from build123d import *

# Parameters (mm, degrees)
SKETCH1_R           = 6.25
SKETCH1_R_2         = 2.6
SKETCH1_R_3         = 6
SKETCH1_W           = 7.5
SKETCH1_H           = 50.316251501
BOSS_EXTRUDE1_DEPTH = 6.5
FILLET1_R           = 10


with BuildPart() as part:
    # Sketch1 → Boss-Extrude1 (new body)
    # profile 1 of 3: a face of its own
    with BuildSketch(Plane(origin=(0, 0, 0), x_dir=(1, 0, 0), z_dir=(0, 1, 0))):
        with Locations((0, 60)):
            Circle(SKETCH1_R)
        with Locations(Location((0, 60, 0), (0, 0, 90))):
            Circle(SKETCH1_R_2, mode=Mode.SUBTRACT)
    # profile 2 of 3: a face of its own
    with BuildSketch(Plane(origin=(0, 0, 0), x_dir=(1, 0, 0), z_dir=(0, 1, 0))):
        Circle(SKETCH1_R_3)
        with Locations(Location((0, 0, 0), (0, 0, 90))):
            Circle(SKETCH1_R_2, mode=Mode.SUBTRACT)
    # profile 3 of 3: a face of its own
    with BuildSketch(Plane(origin=(0, 0, 0), x_dir=(1, 0, 0), z_dir=(0, 1, 0))):
        with Locations((0, 29.84187425)):
            Rectangle(SKETCH1_W, SKETCH1_H)
    extrude(amount=BOSS_EXTRUDE1_DEPTH)

    # Fillet1
    fillet1_edges = [part.edges().sort_by_distance(p)[0] for p in [
        (-3.75, 3.25, -55),
        (3.75, 3.25, -55),
        (3.75, 3.25, -4.683748499),
        (-3.75, 3.25, -4.683748499),
    ]]
    fillet(fillet1_edges, radius=FILLET1_R)


solid = part.part
Work out the finished part from the listing and answer in its coordinate system (mm). A direction names the side the tool comes from. Coordinates: 2 decimals unless noted, no trailing zeros. Write each loop counter-clockwise with the first axis right and the second up, starting at its lowest first coordinate (ties: lowest second). Pieces come first, ordered by that corner, then holes. Notation, with made-up numbers: M -18,41 L 29,41 A24 cw 29,62 Z; hole C 69.25,-25.5 d8. An arc over 180 degrees is marked long. Use one line per item in the form item = value. Start each with the question number.
1. The part is cut by section C-C (y = 1.5). Give the vertices of the cut face in (x, z), plus the area to 3 significant figures.
2. Straight lines are drawn through the part: probe 1 along X at (y, z) = (5, 0); probe 2 along X at (y, z) = (1.5, -60); probe 3 along X at (y, z) = (0.75, -14.5). For each, find the intervals that lie inside material, in ascending order. Write a range as from..to.
3. A tool of negligible diameter and unlimited length cuts with its end or side. For faces 1 (the face through (-0.1, 3.2, -57.4)), 2 (the face through (4.131, 3.296, -54.075)), 3 (the face through (-4.131, 3.296, -54.075)), from which of +Z, -Z, +X, -X, +Y, -Y can it reach the whole face along a straight path? Write none if from no direction.
4. The part is cut by section B-B (x = 0). Give the vertices of the cut face in (y, z), plus the area to 3 significant figures.
5. The part is cut by section A-A (z = -60). Give the vertices of the cut face in (x, y), plus the area to 4 significant figures.
6. The part is cut by section D-D (z = 0). Give the vertices of the cut face in (x, y).
7. The mould has two halves that part along Z. Classify faces 4 (the face through (0, 0, -31)), 5 (the face through (3.75, 3, -29)), 6 (the face through (4.098, 3.296, -5.566)): released by +Z, released by -Z, zero draft, split by the parting line, or undercut.
Evaluation:
q1.outline = M -5.29,-56.67 A6.25 ccw long 5.29,-56.67 A10 cw 3.75,-51.34 L 3.75,-8.18 A10 cw 5.16,-3.07 A6 ccw long -5.16,-3.07 A10 cw -3.75,-8.18 L -3.75,-51.34 A10 cw Z; hole C 0,-60 d5.2; hole C 0,0 d5.2
q1.area = 562 mm^2
q2.probe_1 = -6..-2.6, 2.6..6
q2.probe_2 = -6.25..-2.6, 2.6..6.25
q2.probe_3 = -3.75..3.75
q3.face_1 = +Y, -Y
q3.face_2 = +X, +Y, -Y
q3.face_3 = -X, +Y, -Y
q4.outline = M 0,-66.25 L 6.5,-66.25 L 6.5,-62.6 L 0,-62.6 Z; M 0,-57.4 L 6.5,-57.4 L 6.5,-2.6 L 0,-2.6 Z; M 0,2.6 L 6.5,2.6 L 6.5,6 L 0,6 Z
q4.area = 402 mm^2
q5.outline = M -6.25,0 L -2.6,0 L -2.6,6.5 L -6.25,6.5 Z; M 2.6,0 L 6.25,0 L 6.25,6.5 L 2.6,6.5 Z
q5.area = 47.45 mm^2
q6.outline = M -6,0 L -2.6,0 L -2.6,6.5 L -6,6.5 Z; M 2.6,0 L 6,0 L 6,6.5 L 2.6,6.5 Z
q7.face_4 = zero draft
q7.face_5 = undercut
q7.face_6 = undercut
